Geometry check sheet. Reference: the model listing, model coordinates, mm. A direction names the side the tool comes from. Round coordinates to 2 decimals unless told otherwise and drop trailing zeros. Order: outer loops, then holes, each group sorted by start corner. A loop starts at its lowest first (then second) coordinate and runs counter-clockwise, first axis right, second up. Notation, with made-up numbers: (58.25, 0.25) -> (105.25, 0.25) arc R21 cw to (105.25, 13.25) -> close; hole circle Ø4 at (31.5, 67). An arc over 180 degrees is marked (long way). Answer as a JSON object with one key per item and string values. Group by question number.
Autodesk Inventor part; units mm, degrees
ref_plane "YZ Plane" through (0, 0, 0) normal (1, 0, 0) x (0, 1, 0)
ref_plane "XZ Plane" through (0, 0, 0) normal (0, 1, 0) x (-1, 0, 0)
ref_plane "XY Plane" through (0, 0, 0) normal (0, 0, 1) x (1, 0, 0)
sketch "Sketch1" plane through (0, 0, 0) normal (0, 0, 1) x (1, 0, 0)
  line L0 (-17, 0) -> (-17, 1)
  line L1 (-17, 1) -> (-23, 1)
  line L2 (-23, 1) -> (-23, 5)
  line L3 (-23, 5) -> (-17, 5)
  line L4 (-17, 5) -> (-17, 13)
  line L5 (-17, 13) -> (-23, 13)
  line L6 (-23, 13) -> (-23, 17)
  line L7 (-23, 17) -> (-17, 17)
  line L8 (-17, 17) -> (-17, 24)
  line L9 (-17, 24) -> (0, 24)
  line L10 (0, 24) -> (0, 0)
  line L11 (0, 0) -> (-17, 0)
  dimension "d0" = 4
  dimension "d1" = 17
  dimension "d2" = 1
  dimension "d3" = 24
  dimension "d4" = 6
  dimension "d5" = 8
extrude "Extrusion1" add sketch "Sketch1" along normal blind 50
sketch "Sketch2" plane through (-17, 24, 0) normal (0, 1, 0) x (1, 0, 0)
  line L0 (17, 0) -> (0, 0)
  line L1 (0, 0) -> (0, -50)
  line L2 (0, 0) -> (17, 0)
  line L3 (0, 0) -> (0, 7.1414)
  line L4 (17, 0) -> (17, -50)
  line L5 (0, 0) -> (17, 0)
  arc A0 (17, 0) -> (0, 7.1414) centre (7, 0) ccw
  dimension "d9" = 10
extrude "Extrusion2" add sketch "Sketch2" against normal blind 24
sketch "Sketch3" plane through (-17, 24, 50) normal (0, 1, 0) x (1, 0, 0)
  arc A0 (17, 50) -> (0, 57.1414) centre (7, 50) ccw
  circle A1 centre (7, 50) radius 2
  circle A2 centre (7, 20) radius 2
  line L0 (0, 50) -> (0, 0)
  line L1 (7, 50) -> (7, -10) construction
  line L2 (17, 0) -> (0, 0) construction
  arc A3 (17, 0) -> (-3, 0) centre (7, -10) ccw
  line L3 (17, 50) -> (17, 0) construction
  line L4 (-3, 0) -> (17, 0)
  line L5 (-6, 50) -> (-6, 0) construction
  line L6 (-6, 11.4006) -> (-6, 28.5994)
  arc A4 (-6, 11.4006) -> (-6, 28.5994) centre (-29.9, 20) ccw
  line L7 (7, 20) -> (-4.5, 20) construction
  line L8 (-6, 0) -> (-3.4507, 5.7003)
  line L9 (-3.4507, 5.7003) -> (-6, 11.4006)
  line L10 (-6, 28.5994) -> (-3.7582, 33.612)
  line L11 (-3.7582, 33.612) -> (-6, 38.6246)
  line L12 (-6, 38.6246) -> (-3.4563, 44.3123)
  line L13 (-3.4563, 44.3123) -> (-6, 50)
  line L14 (-6, 0) -> (-6, 11.4006)
  line L15 (-6, 28.5994) -> (-6, 38.6246)
  line L16 (-6, 38.6246) -> (-6, 50)
  dimension "d12" = 4
  dimension "d13" = 60
  dimension "d14" = 11.5
  dimension "d15" = 25.4
extrude "Extrusion3" cut sketch "Sketch3" against normal through all
properties part number "clawGrip" material "Rubber"
Item 1: Mould release check, pull along Y, two halves, no side actions. Record for faces 1 (the flat face through (-19, 17, 25)), 2 (the cylindrical face through (-10, 12, 32)), 3 (the flat face through (-19, 13, 25)), 4 (the flat face through (-8, 0, 20)): pulls with the +Y half, pulls with the -Y half, needs draft (parallel to the pull), parting line crosses it, or undercut.
Item 2: Sectioned sample at C-C, the plane y = 14.75. Enter the section's corners in (x, z), then the cut area to 3 significant figures.
Item 3: Set-up check for faces 5 (the flat face through (-20, 3, 0)), 6 (the flat face through (-21.746, 15.028, 8.571)), 7 (the cylindrical face through (-5.976, 12.168, -9.155)): record each of +Z, -Z, +X, -X, +Y, -Y from which the full face is reachable in a straight line by a thin tool's end or side.
Item 4: Thickness scan on L1, parallel to Z at x = -10, y = 13; L2, parallel to Y at x = -20.75, z = 7; L3, parallel to X at y = 17.5, z = 30. Record the ranges inside material, lowest first.
Item 5: Depth check by flat-ended pin: pin 1 Ø5 at (x, z) = (-20.5, 32.5) entering from +Y; pin 2 Ø5 at (x, z) = (-20.5, 13) entering from -Y; pin 3 Ø3 at (x, z) = (-10, 0) entering from -Y; pin 4 Ø2 at (x, y) = (-7, 18) entering from -Z. Enter the tip coordinate at first touch or a pass-through.
Item 6: Sectioned sample at B-B, the plane z = 30. Enter the section's corners in (x, y).
Item 7: Sectioned sample at A-A, the plane x = -10. Enter the section's corners in (y, z), then the cut area to 3 significant figures.
Item 8: Sectioned sample at D-D, the plane z = 41. Enter the section's corners in (x, y), then the cut area to 3 significant figures.
Result:
{
 "1": {"face 1": "pulls with the +Y half", "face 2": "needs draft", "face 3": "undercut", "face 4": "pulls with the -Y half"},
 "2": {"outline": "(-23, 0) -> (-17, 0) -> (-17, -7.14) arc R10 ccw to (0, 0) -> (0, 50) arc R14.14 cw to (-20, 50) -> (-23, 50) -> (-20.45, 44.3) -> (-23, 38.6) arc R25.4 cw to (-23, 21.4) -> (-20.76, 16.39) -> (-23, 11.38) -> (-20.46, 5.69) -> close; hole circle Ø4 at (-10, 0); hole circle Ø4 at (-10, 30)", "area": "1,150 mm2"},
 "3": {"face 5": "-Z, -X, +Y, -Y", "face 6": "-X, +Y, -Y", "face 7": "-Z, +Y, -Y"},
 "4": {"L1": "z = -10 to -2, 2 to 28, 32 to 45.86", "L2": "y = 1 to 5, 13 to 17", "L3": "x = -17 to -12, -8 to 0"},
 "5": {"pin 1": "stops at y = 17", "pin 2": "stops at y = 1", "pin 3": "passes through", "pin 4": "stops at z = -9.8"},
 "6": {"outline": "(-21.5, 1) -> (-17, 1) -> (-17, 0) -> (-12, 0) -> (-12, 24) -> (-17, 24) -> (-17, 17) -> (-21.5, 17) -> (-21.5, 13) -> (-17, 13) -> (-17, 5) -> (-21.5, 5) -> close; (-8, 0) -> (0, 0) -> (0, 24) -> (-8, 24) -> close"},
 "7": {"outline": "(0, -10) -> (24, -10) -> (24, -2) -> (0, -2) -> close; (0, 2) -> (24, 2) -> (24, 28) -> (0, 28) -> close; (0, 32) -> (24, 32) -> (24, 45.86) -> (0, 45.86) -> close", "area": "1,150 mm2"},
 "8": {"outline": "(-21.93, 1) -> (-17, 1) -> (-17, 0) -> (0, 0) -> (0, 24) -> (-17, 24) -> (-17, 17) -> (-21.93, 17) -> (-21.93, 13) -> (-17, 13) -> (-17, 5) -> (-21.93, 5) -> close", "area": "447 mm2"}
}
